from build123d import *

# Parameters (mm, degrees)
SKETCH1_R           = 9.9
SKETCH1_R_2         = 1.7
BOSS_EXTRUDE2_DEPTH = 2.45
SKETCH2_R           = 4.5
SKETCH2_R_2         = 2.006415725
BOSS_EXTRUDE3_DEPTH = 2.05


with BuildPart() as part:
    # Sketch1 → Boss-Extrude2 (new body)
    with BuildSketch(Plane.XY):
        with Locations((19.5, 0)):
            Circle(SKETCH1_R)
        with Locations((19.5, 0)):
            Circle(SKETCH1_R_2, mode=Mode.SUBTRACT)
        with Locations((12.5, 0)):
            Circle(SKETCH1_R_2, mode=Mode.SUBTRACT)
        with Locations((19.5, 7)):
            Circle(SKETCH1_R_2, mode=Mode.SUBTRACT)
        with Locations((26.5, 0)):
            Circle(SKETCH1_R_2, mode=Mode.SUBTRACT)
        with Locations((19.5, -7)):
            Circle(SKETCH1_R_2, mode=Mode.SUBTRACT)
    extrude(amount=-BOSS_EXTRUDE2_DEPTH)

    # Sketch2 → Boss-Extrude3 (add)
    with BuildSketch(Plane(origin=(0, 0, -2.45), x_dir=(-1, 0, 0), z_dir=(0, 0, -1))):
        with Locations(Location((-19.5, 0, 0), (0, 0, 180))):
            Circle(SKETCH2_R)
        with Locations((-19.5, 0)):
            Circle(SKETCH2_R_2, mode=Mode.SUBTRACT)
    extrude(amount=BOSS_EXTRUDE3_DEPTH)


solid = part.part
The listing builds one solid part. Answer for the finished solid, in the listing's coordinates (mm). A direction names the side the tool comes from. Coordinates: 2 decimals unless noted, no trailing zeros. Loops run counter-clockwise (first coordinate to the right, second up) from the corner with the lowest first, then second, coordinate; pieces in that order, holes last.
1) Find section B-B on y = 7. Write down the section's boundary in (x, z).
2) Flat-ended cylindrical pins translate along their axes: pin 1 Ø2 at (y, z) = (-3.5, -1.5) entering from +X; pin 2 Ø2 at (x, z) = (21.5, -1.5) entering from +Y; pin 3 Ø3 at (x, y) = (19.5, 7) entering from -Z; pin 4 Ø2 at (y, z) = (-3, -3) entering from -X. Find the tip coordinate at first contact, or state that the pin passes through.
3) Find section D-D on x = 12.5. Write down the section's boundary in (y, z).
4) Find the intervals of material crossed by L1, parallel to Y at x = 19.5, z = -1.6; L2, parallel to Z at x = 24.75, y = -3; L3, parallel to Y at x = 19.5, z = -4, in increasing order.
5) Find section A-A on x = 19.5. Write down the section's boundary in (y, z).
6) Find section C-C on z = -2.1. Write down the section's boundary in (x, y).
7) A tool of negligible diameter and unlimited length cuts with its end or side. For faces 1 (the face through (21.07, -0.65, -1.21)), 2 (the face through (17.586, 0.603, -3.461)), from which of +Z, -Z, +X, -X, +Y, -Y can it reach the whole face along a straight path? Write none if from no direction.
8) Determine the mould class of faces 3 (the face through (22, 0, 0)), 4 (the face through (9.61, 0.44, -1.21)), 5 (the face through (14.12, 0.51, -1.21)) for opening direction X: pulls with the +X half, pulls with the -X half, needs draft (parallel to the pull), parting line crosses it, or undercut.
Values:
1. outline: (12.5, -2.45) - (17.8, -2.45) - (17.8, 0) - (12.5, 0) - close; (21.2, -2.45) - (26.5, -2.45) - (26.5, 0) - (21.2, 0) - close
2. pin 1: stops at x = 29.08
2. pin 2: stops at y = 9.85
2. pin 3: passes through
2. pin 4: stops at x = 9.84
3. outline: (-7, -2.45) - (-1.7, -2.45) - (-1.7, 0) - (-7, 0) - close; (1.7, -2.45) - (7, -2.45) - (7, 0) - (1.7, 0) - close
4. L1: y = -9.9 to -8.7, -5.3 to -1.7, 1.7 to 5.3, 8.7 to 9.9
4. L2: z = -2.45 to 0
4. L3: y = -4.5 to -2.01, 2.01 to 4.5
5. outline: (-9.9, -2.45) - (-8.7, -2.45) - (-8.7, 0) - (-9.9, 0) - close; (-5.3, -2.45) - (-4.5, -2.45) - (-4.5, -4.5) - (-2.01, -4.5) - (-2.01, -2.45) - (-1.7, -2.45) - (-1.7, 0) - (-5.3, 0) - close; (1.7, -2.45) - (2.01, -2.45) - (2.01, -4.5) - (4.5, -4.5) - (4.5, -2.45) - (5.3, -2.45) - (5.3, 0) - (1.7, 0) - close; (8.7, -2.45) - (9.9, -2.45) - (9.9, 0) - (8.7, 0) - close
6. outline: circle Ø19.8 at (19.5, 0); hole circle Ø3.4 at (12.5, 0); hole circle Ø3.4 at (19.5, -7); hole circle Ø3.4 at (19.5, 0); hole circle Ø3.4 at (19.5, 7); hole circle Ø3.4 at (26.5, 0)
7. face 1: +Z, -Z
7. face 2: -Z
8. face 3: needs draft
8. face 4: parting line crosses it
8. face 5: undercut
